Verification items for the finished model (mm, model axes). A direction names the side the tool comes from. Coordinates: 2 decimals unless noted, no trailing zeros. Write each loop counter-clockwise with the first axis right and the second up, starting at its lowest first coordinate (ties: lowest second). Pieces come first, ordered by that corner, then holes. Notation, with made-up numbers: (6.25, 5.5) -> (12.25, 5.5) arc R24 cw to (12.25, 29.5) -> close; hole circle Ø4 at (42, 87.25). An arc over 180 degrees is marked (long way). Answer in a Markdown table with one row per item.
```python
from build123d import *

# Parameters (mm, degrees)
F0_R        = 40.5136792868
F0_R_2      = 16.5163542796
F1_DEPTH    = 25.4
F2_W        = 25.4
F2_H        = 8.89
F3_ANGLE    = 180
F4_T2_ANGLE = 180
F4_T4_ANGLE = 180
F4_T6_ANGLE = 180
F5_SIZE     = 3.81


# Not quite as in the source:
# - a fillet or chamfer that OpenCascade refuses, or shapes differently, is made with other operations: its cross-section is extruded or revolved along the edge and cut away or added


with BuildPart() as f1:
    # F0 (on Front) → F1 (new body)
    with BuildSketch(Plane.XZ):
        Circle(F0_R)
        Circle(F0_R_2, mode=Mode.SUBTRACT)
    extrude(amount=F1_DEPTH)

    # F2 (on face) → F3 (revolve)
    with BuildSketch(Plane.XZ.offset(25.4)):
        with Locations((0, 27.305)):
            Rectangle(F2_W, F2_H)
    revolve(axis=Axis((-4.5374315232, -25.4, 0), (1, 0, 0)), revolution_arc=F3_ANGLE)

    # F4: fillet of radius 5.08 on 3 edges, made by hand

    # F4_s1 → F4_t2 (revolve, cut)
    with BuildSketch(Plane.XZ.offset(25.4)):
        with BuildLine():
            ThreePointArc((12.7, 27.94), (11.2121024484, 24.3478975516), (7.62, 22.86))
            Line((7.62, 22.86), (12.7, 22.86))
            Line((12.7, 22.86), (12.7, 27.94))
        make_face()
    revolve(axis=Axis((12.7, -25.4, 0), (1, 0, 0)), revolution_arc=F4_T2_ANGLE, mode=Mode.SUBTRACT)

    # F4_s3 → F4_t4 (revolve, cut)
    with BuildSketch(Plane.XZ.offset(25.4)):
        with BuildLine():
            ThreePointArc((12.7, 26.67), (11.2121024484, 30.2621024484), (7.62, 31.75))
            Line((7.62, 31.75), (12.7, 31.75))
            Line((12.7, 31.75), (12.7, 26.67))
        make_face()
    revolve(axis=Axis((12.7, -25.4, 0), (1, 0, 0)), revolution_arc=F4_T4_ANGLE, mode=Mode.SUBTRACT)

    # F4_s5 → F4_t6 (revolve, cut)
    with BuildSketch(Plane.XZ.offset(25.4)):
        with BuildLine():
            ThreePointArc((-12.7, 26.67), (-11.2121024484, 30.2621024484), (-7.62, 31.75))
            Line((-7.62, 31.75), (-12.7, 31.75))
            Line((-12.7, 31.75), (-12.7, 26.67))
        make_face()
    revolve(axis=Axis((-12.7, -25.4, 0), (1, 0, 0)), revolution_arc=F4_T6_ANGLE, mode=Mode.SUBTRACT)

    # F5
    f5_edges = [f1.edges().sort_by_distance(p)[0] for p in [
        (-40.513679, -25.4, 0),
        (-40.513679, 0, 0),
    ]]
    chamfer(f5_edges, length=F5_SIZE)


solid = f1.part
```
1. Go/stop test with flat-tipped pins: pin 1 (10 mm diameter, centred on y = -26, z = 22.5, fed in from -X); pin 2 (5 mm diameter, centred on y = -19, z = -3, fed in from -X); pin 3 (1.5 mm diameter, centred on x = 1.5, z = -2, fed in from +Y). Record where each tip stops, or that it passes through.
Findings below:
| item | result |
|---|---|
| pin 1 | stops at x = -35.15 |
| pin 2 | stops at x = -40.51 |
| pin 3 | stops at y = -48.09 |
2. Sectioned sample at B-B, the plane x = 0. Record the cut outline in (y, z).
Findings below:
| item | result |
|---|---|
| outline | (-25.4, -36.7) -> (-21.59, -40.51) -> (-3.81, -40.51) -> (0, -36.7) -> (0, -16.52) -> (-25.4, -16.52) -> (-25.4, -22.86) arc R22.86 cw to (-25.4, 22.86) -> (-25.4, 16.52) -> (0, 16.52) -> (0, 36.7) -> (-3.81, 40.51) -> (-21.59, 40.51) -> (-25.4, 36.7) -> (-25.4, 31.75) arc R31.75 ccw to (-25.4, -31.75) -> close |
3. Sectioned sample at A-A, the plane z = 0. Record the cut outline in (x, y) (3 decimals).
Findings below:
| item | result |
|---|---|
| outline | (-40.514, -21.59) -> (-36.704, -25.4) -> (-16.516, -25.4) -> (-16.516, 0) -> (-36.704, 0) -> (-40.514, -3.81) -> close; (-12.7, -52.07) arc R5.08 ccw to (-7.62, -57.15) -> (7.62, -57.15) arc R5.08 ccw to (12.66, -52.705) arc R5.08 ccw to (7.62, -48.26) -> (-12.7, -48.26) -> close; (16.516, -25.4) -> (36.704, -25.4) -> (40.514, -21.59) -> (40.514, -3.81) -> (36.704, 0) -> (16.516, 0) -> close |
4. Sectioned sample at C-C, the plane z = 14. Count the separate pieces of the cut face and the enclosed holes in it, and give its area (3 significant figures).
Findings below:
| item | result |
|---|---|
| separate pieces | 3 |
| enclosed holes | 0 |
| area | 1,700 mm² |
5. Release check for a two-part mould opening along Y. For faces 1 (the face through (-12.7, -49, -2)), 2 (the face through (16, 0, -8)), 3 (the face through (-2.398, -48.254, 0.503)) record: released by +Y, released by -Y, zero draft, split by the parting line, or undercut.
Findings below:
| item | result |
|---|---|
| face 1 | zero draft |
| face 2 | released by +Y |
| face 3 | undercut |
6. Access from +Z, -Z, +X, -X, +Y, -Y to the whole of each face (thin tool, end or side, straight path). Record for faces 4 (the face through (-29.274, -25.215, -22.446)), 5 (the face through (-3.58, -12.522, -16.124)).
Findings below:
| item | result |
|---|---|
| face 4 | -Y |
| face 5 | +Y |
7. Material ranges on probe 1 along Z at (x, y) = (0, -7.25); probe 2 along Z at (x, y) = (-1.5, -20); probe 3 along Y at (x, z) = (-19, -28), recorded low to high. Write a range as from..to.
Findings below:
| item | result |
|---|---|
| probe 1 | z = -40.51..-16.52, 16.52..40.51 |
| probe 2 | z = -40.49..-16.45, 16.45..40.49 |
| probe 3 | y = -25.4..0 |
